Geometry: final body of the model. Coordinates: model frame, mm. A direction names the side the tool comes from. Round coordinates to 2 decimals unless told otherwise and drop trailing zeros. Write each loop counter-clockwise with the first axis right and the second up, starting at its lowest first coordinate (ties: lowest second). Pieces come first, ordered by that corner, then holes. Notation, with made-up numbers: M 87,-35 L 146,-35 A21 cw 146,-22 Z; hole C 21,57.5 d2. An arc over 180 degrees is marked long. Use one line per item in the form item = value. Start each with the question number.
Item 1: Section query A-A (x = 0). Return loops of the section in (y, z), and give its area (3 significant figures).
Item 2: Pin query (flat end, axial travel): pin 1 Ø15.5 at (y, z) = (53, 82.5) entering from -X; pin 2 Ø5 at (y, z) = (31, 11.5) entering from -X; pin 3 Ø5 at (x, z) = (1.5, 83) entering from +Y. Return the tip coordinate at first contact, or that it passes through.
Item 3: Ray query, probe 1 along Y at (x, z) = (0, 6.5); probe 2 along Z at (x, y) = (4.5, -52.5); probe 3 along Y at (x, z) = (32, 5.5). Return the intervals inside material, ascending.
Item 4: Reachability of faces 5 (the flat face through (-8, 50, 59)), 6 (the flat face through (8, 50, 59)), 7 (the flat face through (0, 43.046, 59)) from +Z, -Z, +X, -X, +Y, -Y: full face, straight path, thin tool, end or side. Return the list, or none.
Item 5: Section query B-B (y = 0). Return loops of the section in (x, z).
Item 6: Section query C-C (z = 32.5). Return loops of the section in (x, y), and give its area (3 significant figures).
Item 7: Pull-direction query (Y, two-part tool) for faces 1 (the cylindrical face through (-59.94, 2.64, 4.93)), 2 (the cylindrical face through (56.275, 17.722, 4.944)), 3 (the flat face through (0, 57.046, 59)), 4 (the flat face through (-7, 50, 59)); classes: pulls with the +Y half, pulls with the -Y half, needs draft (parallel to the pull), parting line crosses it, or undercut.
Item 8: Section query D-D (x = 24). Return loops of the section in (y, z), and give its area (3 significant figures).
from build123d import *

# Parameters (mm, degrees)
F0_R     = 60
F1_DEPTH = 10
F2_R     = 40
F3_DEPTH = 10
F4_W     = 16
F4_H     = 14
F5_DEPTH = 100
F6_T     = -1


with BuildPart() as f1:
    # F0 (on Top) → F1 (new body)
    with BuildSketch(Plane.XY):
        Circle(F0_R)
    extrude(amount=F1_DEPTH)

    # F2 (on Top) → F3 (cut)
    with BuildSketch(Plane.XY):
        Circle(F2_R)
    extrude(amount=F3_DEPTH, mode=Mode.SUBTRACT)

    # F4 (on face) → F5 (join)
    with BuildSketch(Plane.XY.offset(10)):
        with Locations((0, 50.0458516181)):
            Rectangle(F4_W, F4_H)
    extrude(amount=F5_DEPTH)

    # F6
    f6_openings = [f1.faces().sort_by_distance(p)[0] for p in [
        (0, 50.045852, 110),
    ]]
    offset(amount=F6_T, openings=f6_openings, kind=Kind.INTERSECTION)


solid = f1.part
Working result:
q1.outline = M -60,0 L -40,0 L -40,10 L -60,10 Z; M 40,0 L 60,0 L 60,10 L 57.05,10 L 57.05,110 L 56.05,110 L 56.05,9 L 59,9 L 59,1 L 41,1 L 41,9 L 44.05,9 L 44.05,110 L 43.05,110 L 43.05,10 L 40,10 Z; hole M -59,1 L -41,1 L -41,9 L -59,9 Z
q1.area = 300 mm²
q2.pin_1 = -8
q2.pin_2 = -52.53
q2.pin_3 = 57.05
q3.probe_1 = -60 to -59, -41 to -40, 40 to 41, 59 to 60
q3.probe_2 = 0 to 1, 9 to 10
q3.probe_3 = -50.75 to -49.57, -25.63 to -24, 24 to 25.63, 49.57 to 50.75
q4.face_5 = +Z, -X, +Y, -Y
q4.face_6 = +Z, +X, +Y, -Y
q4.face_7 = +Z, +X, -X, -Y
q5.outline = M -60,0 L -40,0 L -40,10 L -60,10 Z; M 40,0 L 60,0 L 60,10 L 40,10 Z; hole M -59,1 L -41,1 L -41,9 L -59,9 Z; hole M 41,1 L 59,1 L 59,9 L 41,9 Z
q6.outline = M -8,43.05 L 8,43.05 L 8,57.05 L -8,57.05 Z; hole M -7,44.05 L 7,44.05 L 7,56.05 L -7,56.05 Z
q6.area = 56.0 mm²
q7.face_1 = parting line crosses it
q7.face_2 = undercut
q7.face_3 = pulls with the +Y half
q7.face_4 = undercut
q8.outline = M -54.99,0 L -32,0 L -32,10 L -54.99,10 Z; M 32,0 L 54.99,0 L 54.99,10 L 32,10 Z; hole M -53.9,1 L -33.24,1 L -33.24,9 L -53.9,9 Z; hole M 33.24,1 L 53.9,1 L 53.9,9 L 33.24,9 Z
q8.area = 129 mm²
